Autodesk Inventor part; units mm, degrees
ref_plane "YZ Plane" through (0, 0, 0) normal (1, 0, 0) x (0, 1, 0)
ref_plane "XZ Plane" through (0, 0, 0) normal (0, 1, 0) x (-1, 0, 0)
ref_plane "XY Plane" through (0, 0, 0) normal (0, 0, 1) x (1, 0, 0)
sketch "Sketch1" plane through (0, 0, 0) normal (0, 0, 1) x (1, 0, 0)
  line L0 (-4.5718, -2.6632) -> (-7.5718, -2.6632)
  line L1 (-7.5718, -2.6632) -> (-7.5718, -45.8132)
  line L2 (-7.5718, -45.8132) -> (-4.5718, -45.8132)
  line L3 (-4.5718, -45.8132) -> (-4.5718, -2.6632)
  dimension "d1" = 43.15
  dimension "d2" = 3
revolve "Shoulder" add sketch "Sketch1" angle 360 about axis through (-4.5718, -45.8132, 0) along (0, 1, 0)
sketch "Sketch2" plane through (-4.5718, -2.6632, 0) normal (0, 1, 0) x (1, 0, 0)
  circle A0 centre (0, 0) radius 3
  circle A1 centre (0, 0) radius 2.76
  dimension "d3" = 5.52
extrude "Shoulder_neck" add sketch "Sketch2" along normal blind 1.85 contours A1
sketch "Sketch3" plane through (-4.5718, -0.8132, 0) normal (0, 1, 0) x (1, 0, 0)
  circle A0 centre (0, 0) radius 2.76
  circle A1 centre (0, 0) radius 5.075
  dimension "d6" = 10.15
extrude "Head" add sketch "Sketch3" along normal blind 4.5 contours A0 | A1
sketch "Sketch4" plane through (-4.5718, -45.8132, 0) normal (0, -1, 0) x (1, 0, 0)
  circle A0 centre (0, 0) radius 3
  circle A1 centre (0, 0) radius 1.89
  dimension "d9" = 3.78
extrude "Thread_neck" add sketch "Sketch4" along normal blind 1.8 contours A1
sketch "Sketch5" plane through (-4.5718, -47.6132, 0) normal (0, -1, 0) x (1, 0, 0)
  circle A0 centre (0, 0) radius 1.89
  circle A1 centre (0, 0) radius 2.5
  dimension "d12" = 5
extrude "Thread_shoulder" add sketch "Sketch5" along normal blind 7.7 contours A0 | A1
sketch "Sketch6" plane through (-4.5718, 3.6868, 0) normal (0, 1, 0) x (1, 0, 0)
  circle A0 centre (0, 0) radius 5.075
  circle A1 centre (0, 0) radius 1.5 construction
  line L0 (-1.5, 0.866) -> (-1.5, -0.866)
  line L1 (-1.5, -0.866) -> (0, -1.7321)
  line L2 (0, -1.7321) -> (1.5, -0.866)
  line L3 (1.5, -0.866) -> (1.5, 0.866)
  line L4 (1.5, 0.866) -> (0, 1.7321)
  line L5 (0, 1.7321) -> (-1.5, 0.866)
  dimension "d15" = 3
extrude "Hex" cut sketch "Sketch6" against normal blind 2.4 contours L5 L4 L3 L2 L1 L0
chamfer "Chamfer1" distance 0.24 angle 30 1 edges at (-1.5718, -2.6632, 0) measured on face at (-7.436, -2.6632, -0.4595)
fillet "Fillet1" radius 0.4 1 edges at (-7.3318, -0.8132, 0)
chamfer "Chamfer2" distance 0.3 angle 30 1 edges at (-9.6468, 3.6868, 0) measured on face at (0.4867, 2.1868, 0.4084)
chamfer "Chamfer3" distance 0.4 angle 30 1 edges at (-7.0718, -55.3132, 0) measured on face at (-3.3106, -55.3132, -0.6619)
fillet "Fillet2" radius 0.6 1 edges at (-6.4618, -45.8132, 0)
chamfer "Chamfer7" distance 0.61 angle 30 1 edges at (-7.0718, -47.6132, 0) measured on face at (-2.3177, -47.6132, -0.3502)
thread "Thread"
equation "\"d1\" = Shoulder_length - Shoulder_neck_length"
equation "\"d2\" = 0.5 * Shoulder_diameter"
equation "\"d3\" = Shoulder_neck_dia"
equation "\"d4\" = Shoulder_neck_length"
equation "\"d6\" = Head_diameter"
equation "\"d7\" = Head_height"
equation "\"d9\" = Thread_neck_dia"
equation "\"d10\" = Thread_neck_length"
equation "\"d12\" = Thread_diameter"
equation "\"d13\" = Thread_length - Thread_neck_length"
equation "\"d15\" = Hex_size"
equation "\"d16\" = Hex_length"
equation "\"d18\" = -0.5 * Shoulder_neck_dia + 0.5 * Shoulder_diameter"
equation "\"d64\" = -0.5 * Shoulder_neck_dia + 0.5 * Shoulder_diameter"
equation "\"d21\" = 0.1 * Hex_size"
equation "\"d65\" = 0.1 * Hex_size"
equation "\"d23\" = 0.5 * Thread_pitch"
equation "\"d66\" = 0.5 * Thread_pitch"
equation "\"d25\" = Thread_neck_radius"
equation "\"d60\" = -0.5 * Thread_neck_dia + 0.5 * Thread_diameter"
equation "\"d67\" = -0.5 * Thread_neck_dia + 0.5 * Thread_diameter"
equation "\"Shoulder_diameter\" = 6"
equation "\"Shoulder_length\" = 45"
equation "\"Shoulder_neck_dia\" = 5.52"
equation "\"Thread_diameter\" = 5"
equation "\"Thread_length\" = 9.5"
equation "\"Head_diameter\" = 10.15"
equation "\"Head_height\" = 4.5"
equation "\"Thread_neck_dia\" = 3.78"
equation "\"Hex_size\" = 3"
equation "\"Hex_length\" = 2.4"
equation "\"Thread_pitch\" = 0.8"
equation "\"Shoulder_neck_length\" = 1.85"
equation "\"Thread_neck_length\" = 1.8"
equation "\"Thread_neck_radius\" = 0.6"
properties part number "SCREW, SHOULDER, P, 12.9,  M6X45MM" material "Steel, High Strength Low Alloy"
Can you work these out from the model? Positions are in its coordinate system, mm. A direction names the side the tool comes from. Round coordinates to 2 decimals unless told otherwise and drop trailing zeros. Loops run counter-clockwise (first coordinate to the right, second up) from the corner with the lowest first, then second, coordinate; pieces in that order, holes last.
Item 1: Will these pins go through, and if not, where does the flat tip stop? pin 1 Ø6 at (x, y) = (-6.5, -26.5) entering from -Z; pin 2 Ø6 at (y, z) = (-46, 3) entering from +X; pin 3 Ø4 at (x, y) = (-8.5, -14.5) entering from -Z.
Item 2: If we mould it in two halves opening along Z, with no side actions, what happens to faces 1 (the flat face through (-5.332, 2.504, 1.293)), 2 (the cylindrical face through (-1.575, -24.609, -0.132)), 3 (the flat face through (-4.64, -0.813, 3.31))? For each: +Z half, -Z half, draft (parallel to the pull), parting line (faces both ways), or undercut.
Item 3: Please list where these lines run through material, in increasing order: L1, parallel to Y at x = -5.25, z = 3.5; L2, parallel to Z at x = -5.75, y = -29.5; L3, parallel to X at y = -27, z = 2.75.
Item 4: Suppose I cut it at A-A, the plane y = -8.5. Write out the boundary of the cut face in (x, z).
Item 5: Which directions (+Z, -Z, +X, -X, +Y, -Y) give clear straight access to the entire face, cutting with the end or side of a thin tool? Please do faces 4 (the flat face through (-5.311, 2.504, -1.305)), 5 (the cylindrical face through (-2, -2, 1)), 6 (the flat face through (-5, -55.313, 0)).
Reported:
1. pin 1: stops at z = -3
1. pin 2: stops at x = -1.57
1. pin 3: stops at z = -2.3
2. face 1: undercut
2. face 2: parting line
2. face 3: draft
3. L1: y = -0.81 to 3.69
3. L2: z = -2.76 to 2.76
3. L3: x = -5.77 to -3.37
4. outline: circle Ø6 at (-4.57, 0)
5. face 4: +Y
5. face 5: none
5. face 6: +Z, -Z, +X, -X, -Y
